Read the model definition and answer for the solid it produces. Units are mm, in the model's axes. A direction names the side the tool comes from. Give positions to 0.01 mm unless a question says otherwise; leave off trailing zeros. Order: outer loops, then holes, each group sorted by start corner. A loop starts at its lowest first (then second) coordinate and runs counter-clockwise, first axis right, second up. Notation, with made-up numbers: (86, 35) -> (112, 35) arc R18 cw to (112, 50) -> close; hole circle Ø11 at (24.25, -39). An arc over 180 degrees is marked (long way). Use one line per item in the form item = value.
Autodesk Inventor part; units mm, degrees
ref_plane "YZ Plane" through (0, 0, 0) normal (1, 0, 0) x (0, 1, 0)
ref_plane "XZ Plane" through (0, 0, 0) normal (0, 1, 0) x (-1, 0, 0)
ref_plane "XY Plane" through (0, 0, 0) normal (0, 0, 1) x (1, 0, 0)
sketch "Sketch1" plane through (0, 0, 0) normal (0, 1, 0) x (-1, 0, 0)
  line L0 (-14.3815, 30) -> (14.3815, 30)
  line L1 (14.3815, 30) -> (14.3815, -30)
  line L2 (14.3815, -30) -> (-14.3815, -30)
  line L3 (-14.3815, -30) -> (-14.3815, 30)
  line L4 (-14.3815, 30) -> (14.3815, -30) construction
  line L5 (14.3815, 30) -> (-14.3815, -30) construction
  point P0 (0, 0)
  dimension "d0" = 60
  dimension "d1" = 28.763
extrude "Extrusion1" add sketch "Sketch1" along normal mid plane 5
sketch "Sketch2" plane through (0, 2.5, 0) normal (0, 1, 0) x (1, 0, 0)
  line L0 (-14.3815, -30) -> (14.3815, -30)
  line L1 (-14.3815, -30) -> (-10.3815, -30)
  line L2 (-10.3815, -30) -> (-10.3815, 30)
  line L3 (-10.3815, 30) -> (-14.3815, 30)
  line L4 (-14.3815, 30) -> (-14.3815, -30)
  line L5 (14.3815, 30) -> (-14.3815, 30)
  line L6 (14.3815, -30) -> (10.3815, -30)
  line L7 (10.3815, -30) -> (10.3815, 30)
  line L8 (10.3815, 30) -> (14.3815, 30)
  line L9 (14.3815, 30) -> (14.3815, -30)
  point P0 (0, 0)
  dimension "d4" = 4
  dimension "d5" = 4
extrude "Extrusion2" add sketch "Sketch2" along normal blind 4 contours L4 L3 L2 L0 | L7 L5 L9 L0
sketch "Sketch3" plane through (0, 2.5, 0) normal (0, 1, 0) x (1, 0, 0)
  circle A0 centre (0, 0) radius 1.5875
  dimension "d8" = 3.175
extrude "Extrusion3" add sketch "Sketch3" along normal blind 3
sketch "Sketch4" plane through (0, 2.5, 0) normal (0, 1, 0) x (1, 0, 0)
  line L0 (0, 0) -> (0, -30) construction
  line L1 (0, 0) -> (0, 30) construction
  line L2 (-10.3815, -30) -> (10.3815, -30) construction
  line L3 (10.3815, 30) -> (-10.3815, 30) construction
  point P0 (0, -15)
  point P1 (0, 15)
hole "Hole1" at (0, 2.5, 15) at (0, 2.5, -15) direction (0, -1, 0) diameter 4.305 end through all
sketch "Sketch5" plane through (0, 6.5, 0) normal (0, 1, 0) x (1, 0, 0)
  circle A0 centre (-12.3815, 28) radius 1
  circle A1 centre (-12.3815, -28) radius 1
  circle A2 centre (12.3815, -28) radius 1
  circle A3 centre (12.3815, 28) radius 1
  line L0 (-10.3815, 30) -> (-14.3815, 30)
  line L1 (14.3815, 30) -> (10.3815, 30)
  line L2 (-14.3815, -30) -> (-10.3815, -30)
  point P0 (0, 0)
  point P1 (-12.3815, 30)
  point P2 (12.3815, 30)
  dimension "d18" = 2
  dimension "d19" = 2
  dimension "d20" = 2
extrude "Extrusion4" cut sketch "Sketch5" against normal blind 3
sketch "Sketch7" plane through (0, -2.5, 0) normal (0, -1, 0) x (1, 0, 0)
  line L0 (14.3815, 30) -> (-14.3815, 30)
  line L1 (-14.3815, -10) -> (-11.3815, -10)
  line L2 (-11.3815, -10) -> (-11.3815, 10)
  line L3 (-11.3815, 10) -> (-14.3815, 10)
  line L4 (-14.3815, 10) -> (-14.3815, -10)
  line L5 (-14.3815, 30) -> (-14.3815, -30)
  point P0 (0, 0)
  point P1 (-14.3815, 0)
  dimension "d25" = 3
  dimension "d26" = 20
extrude "Extrusion5" add sketch "Sketch7" along normal blind 20
sketch "Sketch8" plane through (-11.3815, -2.5, 10) normal (1, 0, 0) x (0, 0, -1)
  line L0 (0, 0) -> (0, -20)
  line L1 (20, -20) -> (0, -20)
  point P0 (10, 2.5)
  point P1 (10, -10)
  point P2 (0, -10)
  point P3 (10, -20)
hole "Hole2" at (-11.3815, -12.5, 0) direction (-1, 0, 0) diameter 4.915 end through all
fillet "Fillet1" radius 2 8 edges at (14.3815, 2, 30) (-14.3815, 2, 30) (-14.3815, 2, -30) (14.3815, 2, -30) (-12.8815, -2.5, -10) (-12.8815, -2.5, 10) (-12.8815, -22.5, 10) (-12.8815, -22.5, -10)
equation "\"d5\" = d4"
equation "\"d20\" = d19"
equation "\"BendRadius\" = Thickness"
equation "\"BendReliefWidth\" = Thickness"
equation "\"BendReliefDepth\" = 0.5 * Thickness"
equation "\"CornerReliefSize\" = 4 * Thickness"
equation "\"MinimumRemnant\" = 2 * Thickness"
equation "\"TransitionRadius\" = BendRadius"
equation "\"JacobiRadiusSize\" = Thickness"
equation "\"GapSize\" = Thickness"
properties part number "CameraLinearSupporter"
Item 1: The part is cut by section A-A on z = -15. Give the vertices of the cut face in (x, y), and give its area (3 significant figures).
Checks:
outline = (-14.38, -2.5) -> (-2.15, -2.5) -> (-2.15, 2.5) -> (-10.38, 2.5) -> (-10.38, 6.5) -> (-14.38, 6.5) -> close; (2.15, -2.5) -> (14.38, -2.5) -> (14.38, 6.5) -> (10.38, 6.5) -> (10.38, 2.5) -> (2.15, 2.5) -> close
area = 154 mm²
Item 2: Given pin 1 Ø8.5 at (x, z) = (3, 0) entering from -Y; pin 2 Ø1.8 at (x, z) = (-12.38, -28) entering from +Y; pin 3 Ø16.5 at (x, z) = (-1, -13.5) entering from +Y, each flat-ended and moving along its own axis, determine where each tip first touches the part or whether it passes through.
Checks:
pin_1 = -2.5
pin_2 = 3.5
pin_3 = 2.5
Item 3: Which of the six approach directions +Z, -Z, +X, -X, +Y, -Y give full straight-line access (tool end or side, diameter ignored) to faces 1 (the flat face through (0, 5.5, 0)), 2 (the flat face through (-12, 3.5, 28)), 3 (the flat face through (-13, -12, 10)), 4 (the flat face through (-11.382, -12, -3))?
Checks:
face_1 = +Z, -Z, +Y
face_2 = +Y
face_3 = +Z, +X, -X, -Y
face_4 = +Z, -Z, +X, -Y
Item 4: Straight lines are drawn through the part: L1, parallel to Z at x = 0, y = 0.4; L2, parallel to X at y = 4.1, z = 28; L3, parallel to Z at x = -11.5, y = 4. For each, find the intervals that lie inside material, in ascending order. Write a range as from..to.
Checks:
L1 = -30..-17.15, -12.85..12.85, 17.15..30
L2 = -14.38..-13.38, -11.38..-10.38, 10.38..11.38, 13.38..14.38
L3 = -30..-28.47, -27.53..27.53, 28.47..30
Item 5: The part is cut by section D-D on z = -23.5. Give the vertices of the cut face in (x, y), and give its area (3 significant figures).
Checks:
outline = (-14.38, -2.5) -> (14.38, -2.5) -> (14.38, 6.5) -> (10.38, 6.5) -> (10.38, 2.5) -> (-10.38, 2.5) -> (-10.38, 6.5) -> (-14.38, 6.5) -> close
area = 176 mm²
Item 6: The part is cut by section C-C on y = -12.5. Give the vertices of the cut face in (x, z).
Checks:
outline = (-14.38, -10) -> (-11.38, -10) -> (-11.38, -2.46) -> (-14.38, -2.46) -> close; (-14.38, 2.46) -> (-11.38, 2.46) -> (-11.38, 10) -> (-14.38, 10) -> close
Item 7: Determine the mould class of faces 5 (the cylindrical face through (-12.902, -14.937, 0.32)), 6 (the flat face through (-13, -12, -10)), 7 (the flat face through (12, 3.5, 28)), 8 (the flat face through (0, -2.5, 0)) for opening direction Y: +Y half, -Y half, draft (parallel to the pull), parting line (faces both ways), or undercut.
Checks:
face_5 = undercut
face_6 = draft
face_7 = +Y half
face_8 = -Y half
Item 8: The part is cut by section B-B on x = 0. Give the vertices of the cut face in (y, z), and give its area (3 significant figures).
Checks:
outline = (-2.5, -30) -> (2.5, -30) -> (2.5, -17.15) -> (-2.5, -17.15) -> close; (-2.5, -12.85) -> (2.5, -12.85) -> (2.5, -1.59) -> (5.5, -1.59) -> (5.5, 1.59) -> (2.5, 1.59) -> (2.5, 12.85) -> (-2.5, 12.85) -> close; (-2.5, 17.15) -> (2.5, 17.15) -> (2.5, 30) -> (-2.5, 30) -> close
area = 266 mm²
